Autodesk Inventor part; units mm, degrees
ref_plane "door_to_hinge_XY" through (-177.51, 142.2, 19.53) normal (0, 1, 0) x (1, 0, 0)
ref_plane "door_to_hinge_YZ" through (-177.51, 142.2, 19.53) normal (1, 0, 0) x (0, 0, -1)
ref_plane "door_to_hinge_ZX" through (-177.51, 142.2, 19.53) normal (0, 0, -1) x (0, 1, 0)
sketch "Sketch_2" plane through (0, 0, 0) normal (0, 0, 1) x (1, 0, 0)
  arc A0 (-175, -195) -> (-170, -200) centre (-170, -195) ccw
  line L0 (-170, -200) -> (170, -200)
  arc A1 (170, -200) -> (175, -195) centre (170, -195) ccw
  line L1 (175, -195) -> (175, 195)
  arc A2 (175, 195) -> (170, 200) centre (170, 195) ccw
  line L2 (170, 200) -> (-170, 200)
  arc A3 (-170, 200) -> (-175, 195) centre (-170, 195) ccw
  line L3 (-175, 195) -> (-175, -195)
extrude "Extrusion1" add sketch "Sketch_2" along normal blind 15
sketch "Sketch_3" plane through (0, 0, 0) normal (0, 1, 0) x (-1, 0, 0)
  line L0 (350, -15) -> (350, 30)
  line L1 (350, 30) -> (-350, 30)
  line L2 (-350, 30) -> (-350, -15)
  line L3 (-350, -15) -> (350, -15)
  line L4 (175, 5) -> (175, 15)
  line L5 (175, 15) -> (-175, 15)
  line L6 (-175, 15) -> (-175, 5)
  arc A0 (-175, 5) -> (-170, 0) centre (-170, 5) ccw
  line L7 (-170, 0) -> (170, 0)
  arc A1 (170, 0) -> (175, 5) centre (170, 5) ccw
extrude "Extrusion2" cut sketch "Sketch_3" along normal mid plane 400
sketch "Sketch_4" plane through (0, 0, 0) normal (1, 0, 0) x (0, 1, 0)
  line L0 (400, 30) -> (-400, 30)
  line L1 (-400, 30) -> (-400, -15)
  line L2 (-400, -15) -> (400, -15)
  line L3 (400, -15) -> (400, 30)
  line L4 (200, 15) -> (-200, 15)
  line L5 (-200, 15) -> (-200, 5)
  arc A0 (-200, 5) -> (-195, 0) centre (-195, 5) ccw
  line L6 (-195, 0) -> (195, 0)
  arc A1 (195, 0) -> (200, 5) centre (195, 5) ccw
  line L7 (200, 5) -> (200, 15)
extrude "Extrusion3" cut sketch "Sketch_4" along normal mid plane 350
sketch "Sketch_8" plane through (0, 0, 2) normal (0, 0, 1) x (1, 0, 0)
  arc A0 (-173.25, -194.75) -> (-169.75, -198.25) centre (-169.75, -194.75) ccw
  line L0 (-169.75, -198.25) -> (169.75, -198.25)
  arc A1 (169.75, -198.25) -> (173.25, -194.75) centre (169.75, -194.75) ccw
  line L1 (173.25, -194.75) -> (173.25, 194.75)
  arc A2 (173.25, 194.75) -> (169.75, 198.25) centre (169.75, 194.75) ccw
  line L2 (169.75, 198.25) -> (-169.75, 198.25)
  arc A3 (-169.75, 198.25) -> (-173.25, 194.75) centre (-169.75, 194.75) ccw
  line L3 (-173.25, 194.75) -> (-173.25, -194.75)
extrude "Extrusion4" cut sketch "Sketch_8" along normal blind 15.5
sketch "Sketch_6" plane through (0, 0, 0) normal (0, 0, 1) x (1, 0, 0)
  line L0 (139.4, 11.05) -> (139.4, -11.05)
  line L1 (139.4, -11.05) -> (161.5, -11.05)
  line L2 (161.5, -11.05) -> (161.5, 11.05)
  line L3 (161.5, 11.05) -> (139.4, 11.05)
extrude "Extrusion5" cut sketch "Sketch_6" along normal blind 3
sketch "Sketch_9" plane through (0, 166.75, 0) normal (0, 1, 0) x (1, 0, 0)
  line L0 (-12.5, -3.78) -> (-12.5, -14.5)
  line L1 (-12.5, -14.5) -> (-11, -14.5)
  line L2 (-11, -14.5) -> (-11, -3.78)
  arc A0 (-10.22, -3) -> (-11, -3.78) centre (-10.22, -3.78) ccw
  line L3 (-10.22, -3) -> (10.22, -3)
  arc A1 (11, -3.78) -> (10.22, -3) centre (10.22, -3.78) ccw
  line L4 (11, -3.78) -> (11, -14.5)
  line L5 (11, -14.5) -> (12.5, -14.5)
  line L6 (12.5, -14.5) -> (12.5, -3.78)
  arc A2 (12.5, -3.78) -> (10.22, -1.5) centre (10.22, -3.78) ccw
  line L7 (10.22, -1.5) -> (-10.22, -1.5)
  arc A3 (-10.22, -1.5) -> (-12.5, -3.78) centre (-10.22, -3.78) ccw
extrude "Extrusion6" add sketch "Sketch_9" along normal blind 17.25
sketch "Sketch_10" plane through (0, 0, 0) normal (1, 0, 0) x (0, 1, 0)
  line L0 (188.375, 20.7) -> (162.375, 20.7)
  line L1 (162.375, 20.7) -> (162.375, 8.7)
  line L2 (162.375, 8.7) -> (166.75, 8.7)
  arc A0 (171.05, 13) -> (166.75, 8.7) centre (171.05, 8.7) ccw
  line L3 (171.05, 13) -> (179.7, 13)
  arc A1 (184, 8.7) -> (179.7, 13) centre (179.7, 8.7) ccw
  line L4 (184, 8.7) -> (188.375, 8.7)
  line L5 (188.375, 8.7) -> (188.375, 20.7)
extrude "Extrusion7" cut sketch "Sketch_10" along normal mid plane 30
sketch "Sketch_11" plane through (0, 0, 0) normal (1, 0, 0) x (0, 1, 0)
  circle A0 centre (175.375, 9.2) radius 3.1
extrude "Extrusion8" cut sketch "Sketch_11" along normal mid plane 30
sketch "Sketch_12" plane through (0, 142.2, 0) normal (0, 1, 0) x (1, 0, 0)
  arc A0 (-174.9697, -18.53) -> (-175.1968, -20.9799) centre (-177.51, -19.53) ccw
  line L0 (-175.1968, -20.9799) -> (-172.6754, -16.9572)
  arc A1 (-172.6754, -16.9572) -> (-172.37, -15.895) centre (-174.37, -15.895) ccw
  line L1 (-172.37, -15.895) -> (-172.37, -8.3)
  line L2 (-172.37, -8.3) -> (-173.37, -8.3)
  line L3 (-173.37, -8.3) -> (-173.37, -15.895)
  arc A2 (-173.5227, -16.4261) -> (-173.37, -15.895) centre (-174.37, -15.895) ccw
  line L4 (-173.5227, -16.4261) -> (-176.0442, -20.4488)
  arc A3 (-175.9002, -18.8963) -> (-176.0442, -20.4488) centre (-177.51, -19.53) ccw
  line L5 (-175.9002, -18.8963) -> (-174.9697, -18.53)
extrude "Extrusion9" add sketch "Sketch_12" along normal mid plane 21.75
sketch "Sketch_7" plane through (0, -142.2, 0) normal (0, 1, 0) x (1, 0, 0)
  arc A0 (-174.9697, -18.34) -> (-175.1968, -20.7899) centre (-177.51, -19.34) ccw
  line L0 (-175.1968, -20.7899) -> (-172.6754, -16.7672)
  arc A1 (-172.6754, -16.7672) -> (-172.37, -15.705) centre (-174.37, -15.705) ccw
  line L1 (-172.37, -15.705) -> (-172.37, -8.11)
  line L2 (-172.37, -8.11) -> (-173.37, -8.11)
  line L3 (-173.37, -8.11) -> (-173.37, -15.705)
  arc A2 (-173.5227, -16.2361) -> (-173.37, -15.705) centre (-174.37, -15.705) ccw
  line L4 (-173.5227, -16.2361) -> (-176.0442, -20.2588)
  arc A3 (-175.9002, -18.7063) -> (-176.0442, -20.2588) centre (-177.51, -19.34) ccw
  line L5 (-175.9002, -18.7063) -> (-174.9697, -18.34)
extrude "Extrusion10" add sketch "Sketch_7" along normal mid plane 21.75
ref_plane "door_to_hinge_XY" through (-177.51, 142.2, 19.53) normal (0, 1, 0) x (1, 0, 0)
ref_plane "door_to_hinge_YZ" through (-177.51, 142.2, 19.53) normal (1, 0, 0) x (0, 0, -1)
ref_plane "door_to_hinge_ZX" through (-177.51, 142.2, 19.53) normal (0, 0, -1) x (0, 1, 0)
ref_plane "lock_XY" through (152.45, 0, -7) normal (0, 0, 1) x (1, 0, 0)
ref_plane "lock_YZ" through (152.45, 0, -7) normal (1, 0, 0) x (0, 1, 0)
ref_plane "lock_ZX" through (152.45, 0, -7) normal (0, 1, 0) x (0, 0, 1)
properties part number "jJBDOOR161410HC1"
For this review, take the finished solid that the model builds, in its own axes (mm). A direction names the side the tool comes from. Coordinates: 2 decimals unless noted, no trailing zeros. Write each loop counter-clockwise with the first axis right and the second up, starting at its lowest first coordinate (ties: lowest second). Pieces come first, ordered by that corner, then holes. Notation, with made-up numbers: (73, 62) - (95, 62) arc R28 ccw to (95, 97) - close; hole circle Ø3 at (65.25, 14). An arc over 180 degrees is marked (long way). Answer in a Markdown table with one row per item. Add a question column.
Q1. Draft analysis for pull direction X (two halves, no side actions). For faces 3 (the flat face through (-173.25, 3, 8)), 4 (the flat face through (175, -3, 10)), 5 (the flat face through (-2, 3, 0)), state which applies: +X half, -X half, draft (parallel to the pull), parting line (faces both ways), or undercut.
Q2. We need section C-C, the plane y = 144.5. State the section outline as (x, z) points (3 decimals).
Q3. Tool access review of faces 1 (the flat face through (-2, -200, 10)), 2 (the flat face through (2, 198.25, 8)): name each direction out of +Z, -Z, +X, -X, +Y, -Y from which nothing blocks a thin tool from reaching the whole face with its end or side.
Q4. We need section A-A, the plane x = -56.5. State the section outline as (y, z) points, and give its area (3 significant figures).
Q5. For P1, Ø3, axis at y = 179.5, z = 10.5, coming from the -X side; P2, Ø2, axis at x = -64.5, y = -7, coming from the +Z side; P3, Ø0.6, axis at x = 153, z = 1.5, coming from the -Y side, all flat-tipped, find the tip position at first contact; note any pin that passes through.
Q6. We need section B-B, the plane y = 103.5. State the section outline as (x, z) points, and give its area (3 significant figures).
Q7. For probe 1 along Y at (x, z) = (57.5, 14.75); probe 2 along Y at (x, z) = (11.9, 9.2) (3 decimals); probe 3 along X at (y, z) = (-128, 7.5), list the stretches that pass through material, from the lowest coordinate up.
Answer list:
| question | item | result |
|---|---|---|
| 1 | face 3 | undercut |
| 1 | face 4 | +X half |
| 1 | face 5 | draft |
| 2 | outline | (-176.044, 20.449) - (-173.523, 16.426) arc R1 cw to (-173.37, 15.895) - (-173.37, 15) - (-175, 15) - (-175, 5) arc R5 ccw to (-170, 0) - (170, 0) arc R5 ccw to (175, 5) - (175, 15) - (173.25, 15) - (173.25, 2) - (-173.25, 2) - (-173.25, 8.3) - (-172.37, 8.3) - (-172.37, 15.895) arc R2 ccw to (-172.675, 16.957) - (-175.197, 20.98) arc R2.73 ccw (long way) to (-174.97, 18.53) - (-175.9, 18.896) arc R1.73 cw (long way) to start |
| 3 | face 1 | +Z, -Z, +X, -X, -Y |
| 3 | face 2 | +Z |
| 4 | outline | (-200, 5) arc R5 ccw to (-195, 0) - (195, 0) arc R5 ccw to (200, 5) - (200, 15) - (198.25, 15) - (198.25, 2) - (-198.25, 2) - (-198.25, 15) - (-200, 15) - close |
| 4 | area | 835 mm2 |
| 5 | P1 | stops at x = -175 |
| 5 | P2 | stops at z = 2 |
| 5 | P3 | stops at y = -198.84 |
| 6 | outline | (-175, 5) arc R5 ccw to (-170, 0) - (170, 0) arc R5 ccw to (175, 5) - (175, 15) - (173.25, 15) - (173.25, 2) - (-173.25, 2) - (-173.25, 15) - (-175, 15) - close |
| 6 | area | 735 mm2 |
| 7 | probe 1 | y = -200 to -198.25, 198.25 to 200 |
| 7 | probe 2 | y = -200 to -198.25, 166.779 to 172.275, 178.475 to 183.971, 198.25 to 200 |
| 7 | probe 3 | x = -175 to -173.25, 173.25 to 175 |
